Read the model definition and answer for the solid it produces. Units are mm, in the model's axes. A direction names the side the tool comes from. Coordinates: 2 decimals unless noted, no trailing zeros. Write each loop counter-clockwise with the first axis right and the second up, starting at its lowest first coordinate (ties: lowest second). Pieces come first, ordered by that corner, then holes. Notation, with made-up numbers: M -13,18.25 L 24,18.25 A18 cw 24,38.25 Z; hole C 20,-15.75 d9. An arc over 180 degrees is marked long. Use a Markdown table: item, result. Add a question column.
from build123d import *

# Parameters (mm, degrees)
SKETCH1_W                    = 932.18
SKETCH1_H                    = 57.15
BASE_FLANGE1_DEPTH           = 1.89738
EDGE_FLANGE1_STRIP_W         = 11.65352
EDGE_FLANGE1_STRIP_H         = 1.89738
EDGE_FLANGE1_STRIP_CUT_DEPTH = 932.18
EDGE_FLANGE1_DEPTH           = 932.18
EDGE_FLANGE2_STRIP_W         = 11.65352
EDGE_FLANGE2_STRIP_H         = 1.89738
EDGE_FLANGE2_STRIP_CUT_DEPTH = 932.18
EDGE_FLANGE2_DEPTH           = 932.18
SKETCH12_R                   = 2.4638
CUT_EXTRUDE1_DEPTH           = 471.97413973
FILLET1_R                    = 2.54


# Sheet-metal steps are written as plain solids
with BuildPart() as part:
    # Sketch1 → Base-Flange1 (new body)
    with BuildSketch(Plane(origin=(0, 0, 0), x_dir=(1, 0, 0), z_dir=(0, 1, 0))):
        Rectangle(SKETCH1_W, SKETCH1_H)
    extrude(amount=-BASE_FLANGE1_DEPTH)

    # Edge-Flange1 strip (across the edge) → Edge-Flange1 strip cut (cut)
    with BuildSketch(Plane(origin=(-466.09, 0, 28.575), x_dir=(0, 0, -1), z_dir=(1, 0, 0))):
        with Locations((-1.89738, -0.94869)):
            Rectangle(EDGE_FLANGE1_STRIP_W, EDGE_FLANGE1_STRIP_H)
    extrude(amount=EDGE_FLANGE1_STRIP_CUT_DEPTH, mode=Mode.SUBTRACT)

    # Edge-Flange1 section (across the edge) → Edge-Flange1 (add)
    with BuildSketch(Plane(origin=(-466.09, 0, 28.575), x_dir=(0, 0, -1), z_dir=(1, 0, 0))):
        with BuildLine():
            Line((0, 2.032), (0, 36.20262))
            Line((0, 36.20262), (1.89738, 36.20262))
            Line((1.89738, 36.20262), (1.89738, 2.032))
            ThreePointArc((1.89738, 2.032), (2.492539021, 0.595159021), (3.92938, 0))
            Line((3.92938, 0), (3.92938, -1.89738))
            ThreePointArc((3.92938, -1.89738), (1.150888756, -0.746491244), (0, 2.032))
        make_face()
    extrude(amount=EDGE_FLANGE1_DEPTH)

    # Edge-Flange2 strip (across the edge) → Edge-Flange2 strip cut (cut)
    with BuildSketch(Plane(origin=(466.09, 0, -28.575), x_dir=(0, 0, 1), z_dir=(-1, 0, 0))):
        with Locations((-1.89738, -0.94869)):
            Rectangle(EDGE_FLANGE2_STRIP_W, EDGE_FLANGE2_STRIP_H)
    extrude(amount=EDGE_FLANGE2_STRIP_CUT_DEPTH, mode=Mode.SUBTRACT)

    # Edge-Flange2 section (across the edge) → Edge-Flange2 (add)
    with BuildSketch(Plane(origin=(466.09, 0, -28.575), x_dir=(0, 0, 1), z_dir=(-1, 0, 0))):
        with BuildLine():
            Line((0, 2.032), (0, 36.20262))
            Line((0, 36.20262), (1.89738, 36.20262))
            Line((1.89738, 36.20262), (1.89738, 2.032))
            ThreePointArc((1.89738, 2.032), (2.492539021, 0.595159021), (3.92938, 0))
            Line((3.92938, 0), (3.92938, -1.89738))
            ThreePointArc((3.92938, -1.89738), (1.150888756, -0.746491244), (0, 2.032))
        make_face()
    extrude(amount=EDGE_FLANGE2_DEPTH)

    # Sketch12 → Cut-Extrude1 (cut, through all)
    with BuildSketch(Plane.XY.offset(28.575)):
        with Locations((-458.47, 28.58262)):
            Circle(SKETCH12_R)
        with Locations((-458.47, 9.53262)):
            Circle(SKETCH12_R)
        with Locations((-439.42, 28.58262)):
            Circle(SKETCH12_R)
        with Locations((-439.42, 9.53262)):
            Circle(SKETCH12_R)
    cut_extrude1 = extrude(amount=-CUT_EXTRUDE1_DEPTH, mode=Mode.SUBTRACT)

    # Mirror1: Cut-Extrude1 across plane
    add(cut_extrude1.mirror(Plane(origin=(0, 0, 0), x_dir=(0, 0, 1), z_dir=(1, 0, 0))), mode=Mode.SUBTRACT)

    # Fillet1
    fillet1_edges = [part.edges().sort_by_distance(p)[0] for p in [
        (-466.09, 36.20262, 27.62631),
        (466.09, 36.20262, 27.62631),
        (466.09, 36.20262, -27.62631),
        (-466.09, 36.20262, -27.62631),
    ]]
    fillet(fillet1_edges, radius=FILLET1_R)


solid = part.part
Item 1: Find section A-A on x = 107. Give the vertices of the cut face in (y, z) (3 decimals), then the cut area to 3 significant figures.
Item 2: Find section B-B on z = -15.5. Give the vertices of the cut face in (x, y).
Item 3: Determine the mould class of faces 1 (the flat face through (7, 19, -26.678)), 2 (the flat face through (466.09, -1, 0)), 3 (the flat face through (7, 19, -28.575)) for opening direction Z: pulls with the +Z half, pulls with the -Z half, needs draft (parallel to the pull), parting line crosses it, or undercut.
Item 4: For faces 4 (the flat face through (-7, 19, 26.678)), 5 (the flat face through (-7, -1.897, 0)), determine the directions among +Z, -Z, +X, -X, +Y, -Y from which every point of the face is accessible in a straight line to the end or side of a thin tool.
Item 5: This flat-tipped pin is pushed along its axis until it touches: pin 1 (6.5 mm diameter, centred on x = -439.42, y = 9.53, fed in from -Z) (3 decimals). Where does it stop, or does it pass through?
Item 6: Consider probe 1 along Y at (x, z) = (-458.47, 27.95); probe 2 along Y at (x, z) = (439, -28); probe 3 along Z at (x, y) = (-42.5, 24) (3 decimals). Determine where each line is inside the solid, lowest interval first.
Geometry says:
| question | item | result |
|---|---|---|
| 1 | outline | M -1.897,-24.646 A3.929 ccw 2.032,-28.575 L 36.203,-28.575 L 36.203,-26.678 L 2.032,-26.678 A2.032 cw 0,-24.646 L 0,24.646 A2.032 cw 2.032,26.678 L 36.203,26.678 L 36.203,28.575 L 2.032,28.575 A3.929 ccw -1.897,24.646 Z |
| 1 | area | 241 mm2 |
| 2 | outline | M -466.09,-1.9 L 466.09,-1.9 L 466.09,0 L -466.09,0 Z |
| 3 | face 1 | undercut |
| 3 | face 2 | needs draft |
| 3 | face 3 | pulls with the -Z half |
| 4 | face 4 | +X, -X, +Y |
| 4 | face 5 | +Z, -Z, +X, -X, -Y |
| 5 | pin 1 | stops at z = -28.575 |
| 6 | probe 1 | y = -0.09 to 7.07, 12 to 26.12, 31.05 to 36.2 |
| 6 | probe 2 | y = -0.01 to 7.1, 11.96 to 26.15, 31.01 to 36.2 |
| 6 | probe 3 | z = -28.575 to -26.678, 26.678 to 28.575 |
